from build123d import *

# Parameters (mm, degrees)
BOSS_EXTRUDE1_DEPTH = 15.9
SKETCH2_W           = 24
SKETCH2_H           = 28
BOSS_EXTRUDE2_DEPTH = 12
BOSS_EXTRUDE3_START = -8
SKETCH3_R           = 4
BOSS_EXTRUDE3_DEPTH = 83


with BuildPart() as part:
    # Sketch1 → Boss-Extrude1 (new, symmetric)
    with BuildSketch(Plane.XY):
        Polygon((0, 0), (5.656854249, -5.656854249), (0, -11.313708499), (-5.656854249, -5.656854249), align=None)
    extrude(amount=BOSS_EXTRUDE1_DEPTH, both=True)

    # Sketch2 → Boss-Extrude2 (add, symmetric)
    with BuildSketch(Plane.XY):
        with Locations((0, -22)):
            Rectangle(SKETCH2_W, SKETCH2_H)
    extrude(amount=BOSS_EXTRUDE2_DEPTH, both=True)

    # Sketch3 → Boss-Extrude3 (add)
    with BuildSketch(Plane(origin=(0, 0, 0), x_dir=(1, 0, 0), z_dir=(0, 1, 0)).offset(BOSS_EXTRUDE3_START)):
        with Locations(Location((0, 0, 0), (0, 0, 270))):
            Circle(SKETCH3_R)
    extrude(amount=BOSS_EXTRUDE3_DEPTH)


solid = part.part
Geometry: final body of the model. Coordinates: model frame, mm. A direction names the side the tool comes from. Give positions to 0.01 mm unless a question says otherwise; leave off trailing zeros. Write each loop counter-clockwise with the first axis right and the second up, starting at its lowest first coordinate (ties: lowest second). Pieces come first, ordered by that corner, then holes. Notation, with made-up numbers: (70, -14.75) - (99, -14.75) arc R23 cw to (99, 18.25) - close; hole circle Ø10 at (39, 23). An arc over 180 degrees is marked (long way). Return JSON: item names as keys, results as strings. Group by question number.
1) Section C-C on x = -7.5. Return the cut outline in (y, z), plus the area to 3 significant figures.
2) First-contact query: P1, Ø6, axis at x = -4.5, y = -22, coming from the -Z side; P2, Ø2.5, axis at x = 9, z = -4.5, coming from the +Y side; P3, Ø10, axis at y = 0.5, z = 12.5, coming from the -X side; P4, Ø5, axis at y = 9.5, z = -8, coming from the +X side. Flat tips, straight axial feed; report the tip coordinate or a pass-through.
3) Section B-B on y = -15.5. Return the cut outline in (x, z), plus the area to 3 significant figures.
4) Section A-A on z = 0. Return the cut outline in (x, y).
5) Line query: line 1 (Y direction, x = 4, z = 11); line 2 (Y direction, x = -6, z = 0.5); line 3 (Z direction, x = 6.25, y = -27.5). Output: solid intervals per line, ascending.
6) Mould query, pull axis Y, two halves, no side actions, for faces 1 (the flat face through (0, 75, 0)), 2 (the flat face through (0, -6, -15.9)), 3 (the flat face through (8, -8, 0)). Classes: released by +Y, released by -Y, zero draft, split by the parting line, or undercut.
7) Set-up query: faces 4 (the cylindrical face through (-1.532, 34.923, 3.695)), 5 (the flat face through (5, -5, 0)), 6 (the flat face through (-4.13, -4.13, 0.22)), 7 (the flat face through (12, -22, 0)). Return all of +Z, -Z, +X, -X, +Y, -Y with unobstructed straight access to the full face (end or side cutting, diameter ignored); none if empty.
8) Section D-D on z = -6.5. Return the cut outline in (x, y), plus the area to 3 significant figures.
Filled in:
{
 "1": {"outline": "(-36, -12) - (-8, -12) - (-8, 12) - (-36, 12) - close", "area": "672 mm^2"},
 "2": {"P1": "stops at z = -12", "P2": "stops at y = -8", "P3": "stops at x = -4.5", "P4": "passes through"},
 "3": {"outline": "(-12, -12) - (12, -12) - (12, 12) - (-12, 12) - close", "area": "576 mm^2"},
 "4": {"outline": "(-12, -36) - (12, -36) - (12, -8) - (4, -8) - (4, -7.31) - (5.66, -5.66) - (4, -4) - (4, 75) - (-4, 75) - (-4, -4) - (-5.66, -5.66) - (-4, -7.31) - (-4, -8) - (-12, -8) - close"},
 "5": {"line 1": "y = -36 to -8, -7.31 to -4", "line 2": "y = -36 to -8", "line 3": "z = -12 to 12"},
 "6": {"face 1": "released by +Y", "face 2": "zero draft", "face 3": "undercut"},
 "7": {"face 4": "+Y", "face 5": "+X, +Y", "face 6": "-X, +Y", "face 7": "+Z, -Z, +X, +Y, -Y"},
 "8": {"outline": "(-12, -36) - (12, -36) - (12, -8) - (3.31, -8) - (5.66, -5.66) - (0, 0) - (-5.66, -5.66) - (-3.31, -8) - (-12, -8) - close", "area": "725 mm^2"}
}
